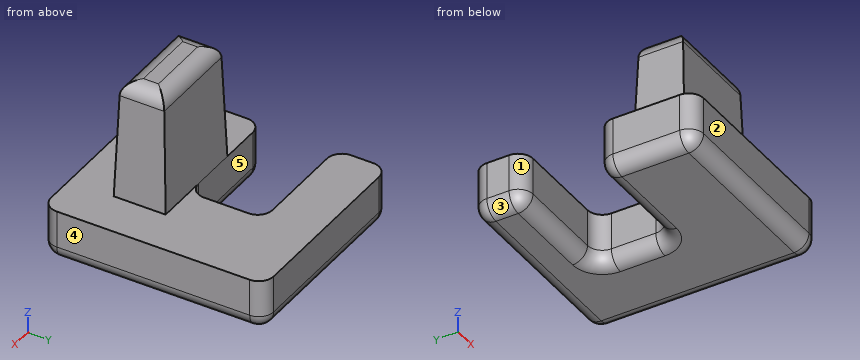
from build123d import *

# Parameters (mm, degrees)
F0_W     = 6.8
F0_H     = 3.5
F1_DEPTH = 8
F1_TAPER = 2
F3_DEPTH = 3.5
F4_R     = 1


with BuildPart() as f1:
    # F0 (on Top) → F1 (new body)
    with BuildSketch(Plane.XY):
        Rectangle(F0_W, F0_H)
    extrude(amount=F1_DEPTH, taper=F1_TAPER)

    # F2 (on face) → F3 (join)
    with BuildSketch(Plane(origin=(0, 0, 0), x_dir=(1, 0, 0), z_dir=(0, 0, -1))):
        with BuildLine():
            Line((3.4, -1.75), (-0.2, -1.75))
            ThreePointArc((-0.2, -1.75), (0.5071067812, -2.0428932188), (0.8, -2.75))
            Line((0.8, -2.75), (0.8, -5.75))
            ThreePointArc((0.8, -5.75), (0.5071067812, -6.4571067812), (-0.2, -6.75))
            Line((-0.2, -6.75), (-3.4, -6.75))
            Line((-3.4, -6.75), (-6.2, -6.75))
            ThreePointArc((-6.2, -6.75), (-6.9071067812, -7.0428932188), (-7.2, -7.75))
            Line((-7.2, -7.75), (-7.2, -9.25))
            ThreePointArc((-7.2, -9.25), (-6.9071067812, -9.9571067812), (-6.2, -10.25))
            Line((-6.2, -10.25), (-3.6740736105, -10.25))
            Line((-3.6740736105, -10.25), (-3.4, -10.25))
            Line((-3.4, -10.25), (5.4, -10.25))
            ThreePointArc((5.4, -10.25), (6.1071067812, -9.9571067812), (6.4, -9.25))
            Line((6.4, -9.25), (6.4, -4.75))
            Line((6.4, -4.75), (6.4, 3.75))
            ThreePointArc((6.4, 3.75), (6.1071067812, 4.4571067812), (5.4, 4.75))
            Line((5.4, 4.75), (-3.4, 4.75))
            Line((-3.4, 4.75), (-6.2, 4.75))
            ThreePointArc((-6.2, 4.75), (-6.9071067812, 4.4571067812), (-7.2, 3.75))
            Line((-7.2, 3.75), (-7.2, -0.75))
            ThreePointArc((-7.2, -0.75), (-6.9071067812, -1.4571067812), (-6.2, -1.75))
            Line((-6.2, -1.75), (-3.4, -1.75))
            Line((-3.4, -1.75), (-3.4, 1.75))
            Line((-3.4, 1.75), (3.4, 1.75))
            Line((3.4, 1.75), (3.4, -1.75))
        make_face()
        Polygon((-3.4, -1.75), (-0.2, -1.75), (3.4, -1.75), (3.4, 1.75), (-3.4, 1.75), align=None)
    extrude(amount=F3_DEPTH)

    # F4
    f4_edges = [f1.edges().sort_by_distance(p)[0] for p in [
        (-0.4, 10.25, -3.5),
        (0, 1.470634, 8),
        (0, -1.470634, 8),
        (-3.120634, 0, 8),
        (3.120634, 0, 8),
    ]]
    fillet(f4_edges, radius=F4_R)


solid = f1.part
Here's how the part is built. I have some questions about the finished solid (model axes, mm). Face numbers are marked on the shaded views. A direction names the side the tool comes from. Round coordinates to 2 decimals unless told otherwise and drop trailing zeros. Order: outer loops, then holes, each group sorted by start corner. A loop starts at its lowest first (then second) coordinate and runs counter-clockwise, first axis right, second up. Notation, with made-up numbers: M 88,1.25 L 139,1.25 A24 ccw 139,23.25 Z; hole C -19.5,-4 d1. An arc over 180 degrees is marked long. Return JSON: item names as keys, results as strings. Group by question number.
1. Please list where these lines run through material, in increasing order: probe 1 along Z at (x, y) = (2.5, 6.75); probe 2 along X at (y, z) = (5, -1); probe 3 along X at (y, z) = (9.5, -1.5).
2. On a 3-axis mill with a long thin cutter (end or side, diameter ignored), from which of +Z, -Z, +X, -X, +Y, -Y can I reach the whole of each face in a straight line? I mean the marked faces 4 and 5. Say none if no direction works.
3. I'm going to push flat-ended pins straight in: pin 1 Ø2 at (y, z) = (1, 1.5) entering from -X; pin 2 Ø3 at (y, z) = (5, -1) entering from -X; pin 3 Ø1.5 at (x, z) = (-2, 1.5) entering from +Y. Where does each tip first touch, or does it pass through?
4. If we section it at A-A on x = -0.75: List the corners of the cut face in (y, z) for me, then the cut area to 3 significant figures.
5. If we section it at D-D on x = -5: List the corners of the cut face in (y, z) for me, then the cut area to 3 significant figures.
6. If we section it at B-B on z = -2.25: List the corners of the cut face in (x, y) for me, then the cut area to 3 significant figures.
7. If we mould it in two halves opening along Y, with no side actions, what happens to the marked faces 1, 2 and 3? For each: pulls with the +Y half, pulls with the -Y half, needs draft (parallel to the pull), parting line crosses it, or undercut.
8. If we section it at C-C on y = 5: List the corners of the cut face in (x, z) for me.
Reply:
{
 "1": {"probe 1": "-3.5 to 0", "probe 2": "0.8 to 6.4", "probe 3": "-7.17 to 6.37"},
 "2": {"face 4": "+Z, -Z, +X, +Y, -Y", "face 5": "+Z, -Z, -X"},
 "3": {"pin 1": "x = -3.38", "pin 2": "x = 0.46", "pin 3": "y = 1.72"},
 "4": {"outline": "M -4.75,-2.5 A1 ccw -3.75,-3.5 L 0.75,-3.5 A1 ccw 1.75,-2.5 L 1.75,0 L 1.5,7.03 A1 ccw 0.5,8 L -0.5,8 A1 ccw -1.5,7.03 L -1.75,0 L -4.75,0 Z; M 6.75,-2.5 A1 ccw 7.75,-3.5 L 9.25,-3.5 A1 ccw 10.25,-2.5 L 10.25,0 L 6.75,0 Z", "area": "59.5 mm^2"},
 "5": {"outline": "M -4.75,-2.5 A1 ccw -3.75,-3.5 L 0.75,-3.5 A1 ccw 1.75,-2.5 L 1.75,0 L -4.75,0 Z; M 6.75,-2.5 A1 ccw 7.75,-3.5 L 9.25,-3.5 A1 ccw 10.25,-2.5 L 10.25,0 L 6.75,0 Z", "area": "34.1 mm^2"},
 "6": {"outline": "M -7.2,-3.75 A1 ccw -6.2,-4.75 L 5.4,-4.75 A1 ccw 6.4,-3.75 L 6.4,9.25 A1 ccw 5.4,10.25 L -6.2,10.25 A1 ccw -7.2,9.25 L -7.2,7.75 A1 ccw -6.2,6.75 L -0.2,6.75 A1 cw 0.8,5.75 L 0.8,2.75 A1 cw -0.2,1.75 L -6.2,1.75 A1 ccw -7.2,0.75 Z", "area": "163 mm^2"},
 "7": {"face 1": "undercut", "face 2": "pulls with the -Y half", "face 3": "needs draft"},
 "8": {"outline": "M 0.8,-2.5 A1 ccw 1.8,-3.5 L 5.4,-3.5 A1 ccw 6.4,-2.5 L 6.4,0 L 0.8,0 Z"}
}
